Check sheet for the modelled part. Datum: model origin and axes. Units: mm. A direction names the side the tool comes from. Round coordinates to 2 decimals unless told otherwise and drop trailing zeros. Write each loop counter-clockwise with the first axis right and the second up, starting at its lowest first coordinate (ties: lowest second). Pieces come first, ordered by that corner, then holes. Notation, with made-up numbers: (5.5, 1.25) -> (28.5, 1.25) arc R14 ccw to (28.5, 21.25) -> close; hole circle Ø2 at (-38.5, 42). An arc over 180 degrees is marked (long way). One line per item, written item: value.
from build123d import *

# Parameters (mm, degrees)
BOSS_EXTRUDE1_DEPTH = 16
CHAMFER1_SIZE       = 2
SKETCH2_R           = 2.25
CUT_EXTRUDE1_DEPTH  = 16
CUT_EXTRUDE2_DEPTH  = 16
SKETCH5_R           = 1.35
CUT_EXTRUDE3_DEPTH  = 16
CHAMFER3_SIZE       = 5


with BuildPart() as part:
    # Sketch1 → Boss-Extrude1 (new body)
    with BuildSketch(Plane.XY):
        Polygon((0, 0), (0, 13), (54, 13), (54, 0), (45, 0), (45, 10.2), (9, 10.2), (9, 0), align=None)
    extrude(amount=BOSS_EXTRUDE1_DEPTH)

    # Chamfer1
    chamfer1_edges = [part.edges().sort_by_distance(p)[0] for p in [
        (0, 0, 8),
        (54, 0, 8),
        (45, 0, 8),
        (9, 0, 8),
    ]]
    chamfer(chamfer1_edges, length=CHAMFER1_SIZE)

    # Sketch2 → Cut-Extrude1 (cut)
    with BuildSketch(Plane.XY.offset(16)):
        with Locations((4.5, 5)):
            Circle(SKETCH2_R)
        with Locations((49.5, 5)):
            Circle(SKETCH2_R)
    extrude(amount=-CUT_EXTRUDE1_DEPTH, mode=Mode.SUBTRACT)

    # Sketch3 → Cut-Extrude2 (cut)
    with BuildSketch(Plane.XY.offset(16)):
        with BuildLine():
            Line((2.534938179, 3.904083927), (6.465061821, 3.904083927))
            ThreePointArc((6.465061821, 3.904083927), (6.1, 2.5), (6.465061821, 1.095916073))
            Line((6.465061821, 1.095916073), (7, 0))
            Line((7, 0), (2, 0))
            Line((2, 0), (2.534938179, 1.095916073))
            ThreePointArc((2.534938179, 1.095916073), (2.9, 2.5), (2.534938179, 3.904083927))
        make_face()
        with BuildLine():
            Line((4.1, 9.052786405), (4.1, 6.794596967))
            Line((4.1, 6.794596967), (4.9, 6.794596967))
            Line((4.9, 6.794596967), (4.9, 9.052786405))
            ThreePointArc((4.9, 9.052786405), (4.5, 10.1), (4.1, 9.052786405))
        make_face()
    cut_extrude2 = extrude(amount=-CUT_EXTRUDE2_DEPTH, mode=Mode.SUBTRACT)

    # Mirror1: Cut-Extrude2 across plane
    add(cut_extrude2.mirror(Plane(origin=(27, 0, 0), x_dir=(0, 0, 1), z_dir=(1, 0, 0))), mode=Mode.SUBTRACT)

    # Sketch5 → Cut-Extrude3 (cut)
    with BuildSketch(Plane(origin=(0, 13, 0), x_dir=(1, 0, 0), z_dir=(0, 1, 0))):
        with Locations(Location((24.4, -2.96, 0), (0, 0, 270))):
            Circle(SKETCH5_R)
        with Locations(Location((43.5, -2.96, 0), (0, 0, 270))):
            Circle(SKETCH5_R)
        with BuildLine():
            Line((20.7, -5.1), (20.7, -10.9))
            ThreePointArc((20.7, -10.9), (18.5, -13.1), (16.3, -10.9))
            Line((16.3, -10.9), (16.3, -5.1))
            ThreePointArc((16.3, -5.1), (18.5, -2.9), (20.7, -5.1))
        make_face()
        with BuildLine():
            Line((29.7, -7.3), (38.7, -7.3))
            ThreePointArc((38.7, -7.3), (40.9, -9.5), (38.7, -11.7))
            Line((38.7, -11.7), (29.7, -11.7))
            ThreePointArc((29.7, -11.7), (27.5, -9.5), (29.7, -7.3))
        make_face()
    extrude(amount=-CUT_EXTRUDE3_DEPTH, mode=Mode.SUBTRACT)

    # Chamfer3
    chamfer3_edges = [part.edges().sort_by_distance(p)[0] for p in [
        (0, 13, 8),
        (54, 13, 8),
    ]]
    chamfer(chamfer3_edges, length=CHAMFER3_SIZE)


solid = part.part
Item 1: Sectioned sample at B-B on x = 43. Enter the section's corners in (y, z), and give its area (3 significant figures).
Answer:
outline: (10.2, 0) -> (13, 0) -> (13, 1.71) -> (10.2, 1.71) -> close; (10.2, 4.21) -> (13, 4.21) -> (13, 16) -> (10.2, 16) -> close
area: 37.8 mm^2
Item 2: Thickness scan on line 1 (Z direction, x = 37, y = 12); line 2 (X direction, y = 9.5, z = 11); line 3 (X direction, y = 1, z = 1). Record the ranges inside material, lowest first.
Answer:
line 1: z = 0 to 7.3, 11.7 to 16
line 2: x = 1.5 to 3.9, 5.1 to 9, 45 to 48.9, 50.1 to 52.5
line 3: x = 1 to 2.49, 6.51 to 8, 46 to 47.49, 51.51 to 53
Item 3: Mould release check, pull along Z, two halves, no side actions. Record for faces 4 (the flat face through (27.1, 10.4, 0)), 5 (the flat face through (49.9, 8, 8)), 6 (the flat face through (27.1, 10.4, 16)), 7 (the cylindrical face through (42.18, 11.62, 2.67)): pulls with the +Z half, pulls with the -Z half, needs draft (parallel to the pull), parting line crosses it, or undercut.
Answer:
face 4: pulls with the -Z half
face 5: needs draft
face 6: pulls with the +Z half
face 7: undercut
Item 4: Sectioned sample at C-C on y = 11.5. Enter the section's corners in (x, z), and give its area (3 significant figures).
Answer:
outline: (3.5, 0) -> (50.5, 0) -> (50.5, 16) -> (3.5, 16) -> close; hole (16.3, 5.1) arc R2.2 ccw to (20.7, 5.1) -> (20.7, 10.9) arc R2.2 ccw to (16.3, 10.9) -> close; hole circle Ø2.7 at (24.4, 2.96); hole (29.7, 7.3) -> (38.7, 7.3) arc R2.2 ccw to (38.7, 11.7) -> (29.7, 11.7) arc R2.2 ccw to start; hole circle Ø2.7 at (43.5, 2.96)
area: 645 mm^2
Item 5: Depth check by flat-ended pin: P1, Ø2, axis at x = 7.5, z = 2, coming from the -Y side; P2, Ø2, axis at y = 11.5, z = 8.5, coming from the -X side; P3, Ø1.6, axis at x = 43.5, z = 2.96, coming from the +Y side; P4, Ø1.4, axis at y = 11.5, z = 8.5, coming from the +X side. Enter the tip coordinate at first touch or a pass-through.
Answer:
P1: stops at y = 0
P2: stops at x = 2.5
P3: passes through
P4: stops at x = 51.2
Item 6: Tool access check on faces 1 (the flat face through (49.1, 8, 8)), 2 (the flat face through (34, 12, 11.7)), 3 (the cylindrical face through (51.1, 2.5, 8.1)). Record the directions out of +Z, -Z, +X, -X, +Y, -Y that give a thin tool (end or side, any length) a straight path to the whole face; none if there is none.
Answer:
face 1: +Z, -Z, -Y
face 2: +Y, -Y
face 3: +Z, -Z
